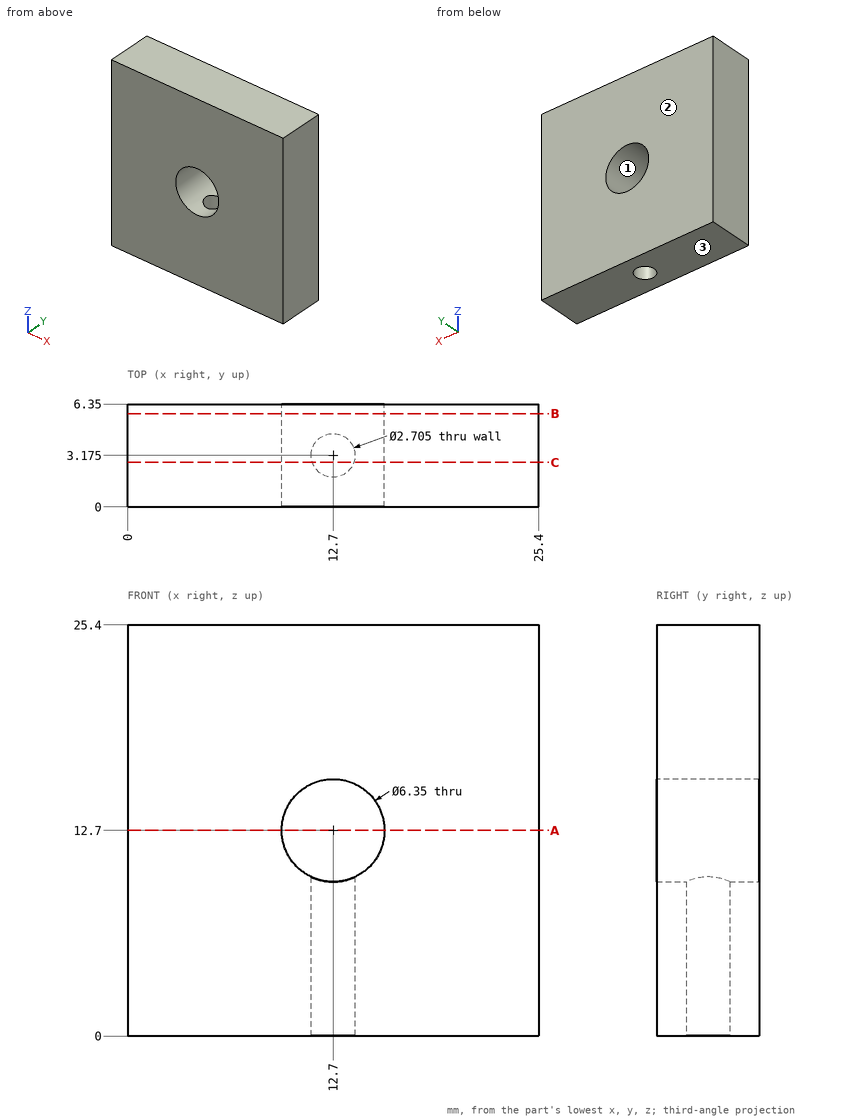
Study the drawing (mm; zero at the part's minimum x, y, z) and answer. Give positions to 0.01 mm unless a question says otherwise; leave off trailing zeros. Write each loop counter-clockwise with the first axis right and the second up, starting at its lowest first coordinate (ties: lowest second). Pieces come first, ordered by that corner, then holes. Notation, with made-up numbers: (-22, 74) - (-11, 74) arc R5 ccw to (-11, 82) - close; hole circle Ø4 at (32.5, 61.25). An arc over 180 degrees is marked (long way). Use CSV: the item, a comma, the result in double quotes. Start each with the question number.
(1) Find section A-A (z = 12.7). Give the vertices of the cut face in (x, y) (3 decimals), plus the area to 3 significant figures.
(2) Find section B-B (y = 5.75). Give the vertices of the cut face in (x, z) (3 decimals).
(3) Consider line 1 along X through (y, z) = (4.25, 12.75); line 2 along Z through (x, y) = (12.7, 5.25) (3 decimals); line 3 along Y through (x, z) = (12.7, 2.5). Determine where each line is inside the solid, lowest interval first.
(4) Given P1, Ø2, axis at y = 2, z = 15.5, coming from the -X side; P2, Ø2, axis at x = 12.7, y = 3.175, coming from the -Z side, each flat-ended and moving along its own axis, determine where each tip first touches the part or whether it passes through.
(5) Determine the mould class of the marked faces 1, 2 and 3 for opening direction Z: +Z half, -Z half, draft (parallel to the pull), parting line (faces both ways), or undercut.
(6) Find section C-C (y = 2.75). Give the vertices of the cut face in (x, z) (3 decimals).
Findings below:
1,outline,"(0, 0) - (9.525, 0) - (9.525, 6.35) - (0, 6.35) - close; (15.875, 0) - (25.4, 0) - (25.4, 6.35) - (15.875, 6.35) - close"
1,area,"121 mm2"
2,outline,"(0, 0) - (25.4, 0) - (25.4, 25.4) - (0, 25.4) - close; hole circle Ø6.35 at (12.7, 12.7)"
3,line 1,"0 to 9.53, 15.87 to 25.4"
3,line 2,"0 to 9.525, 15.875 to 25.4"
3,line 3,"0 to 1.82, 4.53 to 6.35"
4,P1,"x = 0"
4,P2,"z = 15.71"
5,face 1,"undercut"
5,face 2,"draft"
5,face 3,"-Z half"
6,outline,"(0, 0) - (11.416, 0) - (11.416, 9.796) arc R3.175 cw (long way) to (13.984, 9.796) - (13.984, 0) - (25.4, 0) - (25.4, 25.4) - (0, 25.4) - close"
